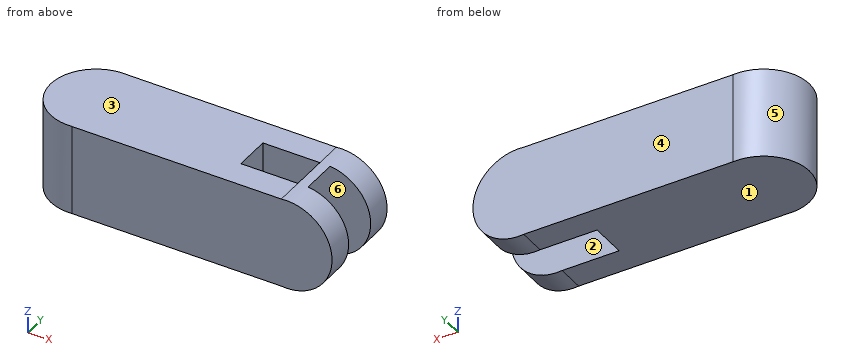
```python
from build123d import *

# Parameters (mm, degrees)
F0_W     = 76.2
F0_H     = 31.75
F1_DEPTH = 31.75
F2_R     = 15.976301
F3_DEPTH = 31.75
F4_R     = 15.912234
F5_DEPTH = 31.75
F6_W     = 38.1
F6_H     = 12.7
F7_DEPTH = 31.852301


with BuildPart() as f1:
    # F0 (on Front) → F1 (new body)
    with BuildSketch(Plane.XZ):
        with Locations((6.312966, 2.627858)):
            Rectangle(F0_W, F0_H)
    extrude(amount=F1_DEPTH)

    # F2 (on face) → F3 (join)
    with BuildSketch(Plane.XZ.offset(31.75)):
        with Locations((44.412966, 2.627858)):
            Circle(F2_R)
    extrude(amount=-F3_DEPTH)

    # F4 (on face) → F5 (join)
    with BuildSketch(Plane.XY.offset(18.502858)):
        with Locations((-31.787034, -15.875)):
            Circle(F4_R)
    extrude(amount=-F5_DEPTH)

    # F6 (on face) → F7 (cut, through all)
    with BuildSketch(Plane.XY.offset(18.502858)):
        with Locations((41.720474, -15.823372)):
            Rectangle(F6_W, F6_H)
    extrude(amount=-F7_DEPTH, mode=Mode.SUBTRACT)


solid = f1.part
```
The listing builds one solid part. Answer for the finished solid, in the listing's coordinates (mm). Face numbers are marked on the shaded views. A direction names the side the tool comes from. Coordinates: 2 decimals unless noted, no trailing zeros. Write each loop counter-clockwise with the first axis right and the second up, starting at its lowest first coordinate (ties: lowest second). Pieces come first, ordered by that corner, then holes. Notation, with made-up numbers: (57, 66) -> (94, 66) arc R16 cw to (94, 84) -> close; hole circle Ø2 at (49.5, 15). An arc over 180 degrees is marked (long way). Write each question's results on one line, items separated by ' | '. Start each with the question number.
1) A cutting plane is placed at C-C (y = -16). Determine the outline of the cut face in (x, z), then the cut area to 3 significant figures.
2) For a pull along Y with two mould halves and no side action, classify the marked faces 4, 5 and 6 as +Y half, -Y half, draft (parallel to the pull), parting line (faces both ways), or undercut.
3) A cutting plane is placed at A-A (x = 26). Determine the outline of the cut face in (y, z).
4) Straight lines are drawn through the part: probe 1 along Y at (x, z) = (48, 1.5); probe 2 along Z at (x, y) = (-4.5, -3.5). For each, find the intervals that lie inside material, in ascending order.
5) A cutting plane is placed at D-D (x = 50.5). Determine the outline of the cut face in (y, z), then the cut area to 3 significant figures.
6) A tool of negligible diameter and unlimited length cuts with its end or side. For the marked faces 1, 2 and 3, from which of +Z, -Z, +X, -X, +Y, -Y can it reach the whole face along a straight path? Write none if from no direction.
7) Flat-ended cylindrical pins translate along their axes: pin 1 Ø9.5 at (x, y) = (20, -9.5) entering from +Z; pin 2 Ø5 at (y, z) = (-10, 8) entering from +X; pin 3 Ø16 at (x, z) = (50.5, -0.5) entering from -Y. Find the tip coordinate at first contact, or state that the pin passes through.
8) A cutting plane is placed at B-B (z = -4.5). Determine the outline of the cut face in (x, y) (3 decimals).
Values follow:
1) outline: (-47.7, -13.25) -> (22.67, -13.25) -> (22.67, 18.5) -> (-47.7, 18.5) -> close; (42.62, 18.5) -> (46.21, 18.5) arc R15.98 ccw to start | area: 2,230 mm²
2) face 4: +Y half | face 5: parting line | face 6: undercut
3) outline: (-31.75, -13.25) -> (-22.17, -13.25) -> (-22.17, 18.5) -> (-31.75, 18.5) -> close; (-9.47, -13.25) -> (0, -13.25) -> (0, 18.5) -> (-9.47, 18.5) -> close
4) probe 1: -31.75 to -22.17, -9.47 to 0 | probe 2: -13.25 to 18.5
5) outline: (-31.75, -12.14) -> (-22.17, -12.14) -> (-22.17, 17.4) -> (-31.75, 17.4) -> close; (-9.47, -12.14) -> (0, -12.14) -> (0, 17.4) -> (-9.47, 17.4) -> close | area: 563 mm²
6) face 1: -Z, -X, +Y, -Y | face 2: -Z, +X | face 3: +Z, -X, +Y, -Y
7) pin 1: z = 18.5 | pin 2: x = 60.12 | pin 3: y = -31.75
8) outline: (-30.699, -31.75) -> (58.711, -31.75) -> (58.711, -22.173) -> (22.67, -22.173) -> (22.67, -9.473) -> (58.711, -9.473) -> (58.711, 0) -> (-30.699, 0) arc R15.912 ccw (long way) to start
